```python
from build123d import *

# Parameters (mm, degrees)
F0_W      = 508
F0_H      = 254
F1_DEPTH  = 2.54
F3_DEPTH  = 203.2
F5_DEPTH  = 203.2
F6_W      = 76.2
F6_H      = 155.0987733221
F7_DEPTH  = 25.4
F9_DEPTH  = 76.2
F10_W     = 7.7724000598
F10_H     = 15.7987965533
F10_H_2   = 18.846809864
F10_H_3   = 19.9136117986
F11_DEPTH = 76.2
F12_W     = 38.3358041449
F12_H     = 114.723880429
F13_DEPTH = 25.4
F14_R     = 12.7
F15_DEPTH = 50.8
F16_W     = 76.2
F16_H     = 165.1
F17_DEPTH = 25.4
F18_W     = 254
F18_H     = 8.89
F18_W_2   = 139.9702800131
F19_DEPTH = 38.1


with BuildPart() as f1:
    # F0 (on Top) → F1 (new body)
    with BuildSketch(Plane.XY):
        with Locations((1.6115792096, -65.0062360242)):
            Rectangle(F0_W, F0_H)
    extrude(amount=F1_DEPTH)

    # F2 (on face) → F3 (join)
    with BuildSketch(Plane.XY.offset(2.54)):
        Polygon((-252.3884207904, 61.9937639758), (-252.3884207904, -192.0062360242), (-249.8484207904, -192.0062360242), (-249.8484207904, 59.4537639758), (255.6115792096, 59.4537639758), (255.6115792096, 61.9937639758), align=None)
    extrude(amount=F3_DEPTH)

    # F4 (on face) → F5 (join)
    with BuildSketch(Plane.XY.offset(2.54)):
        Polygon((-249.8484207904, -189.4662360242), (-249.8484207904, -192.0062360242), (-122.8484207904, -192.0062360242), (-139.9702800131, 59.4537639758), (-142.5102800131, 59.4537639758), (-125.5613688634, -189.4662360242), align=None)
    extrude(amount=F5_DEPTH)

    # F6 (on face) → F7 (cut)
    with BuildSketch(Plane(origin=(-135.2948289897, -9.2121968326, 0), x_dir=(-0.0679324996, 0.9976899195, 0), z_dir=(0.9976899195, 0.0679324996, 0))):
        with Locations((-38.1, 80.0893866611)):
            Rectangle(F6_W, F6_H)
    extrude(amount=-F7_DEPTH, mode=Mode.SUBTRACT)

    # F8 (on face) → F9 (join)
    with BuildSketch(Plane.XY.offset(2.54)):
        Polygon((-78.7540227175, -182.3542267084), (-43.1940241251, -182.3542267084), (-7.6340255328, -182.3542267084), (-28.2588265836, -108.7450310588), (-43.1940241251, -108.7450310588), (-58.1292216666, -108.7450310588), align=None)
    extrude(amount=F9_DEPTH)

    # F10 (on face) → F11 (join)
    with BuildSketch(Plane.XY.offset(2.54)):
        with Locations((-1.2078255029, -83.0656343008)):
            Rectangle(F10_W, F10_H)
        with Locations((-1.2078255029, -132.7480375767)):
            Rectangle(F10_W, F10_H_2)
        with Locations((-1.2078255029, -179.5094301249)):
            Rectangle(F10_W, F10_H_3)
        with Locations((29.1197744374, -83.0656343008)):
            Rectangle(F10_W, F10_H)
        with Locations((29.1197744374, -132.7480375767)):
            Rectangle(F10_W, F10_H_2)
        with Locations((29.1197744374, -179.5094301249)):
            Rectangle(F10_W, F10_H_3)
        Polygon((86.0411706011, -108.7450310588), (56.1707755181, -108.7450310588), (35.5459744672, -182.3542267084), (106.665971652, -182.3542267084), align=None)
    extrude(amount=F11_DEPTH)

    # F12 (on face) → F13 (join)
    with BuildSketch(Plane.XY.offset(78.74)):
        with Locations((14.0738765397, -132.5281762387)):
            Rectangle(F12_W, F12_H)
    extrude(amount=-F13_DEPTH)

    # F14 (on face) → F15 (join)
    with BuildSketch(Plane.XY.offset(2.54)):
        with Locations((-43.1940241251, -90.2538299561)):
            Circle(F14_R)
        with Locations((71.1059730596, -90.2538299561)):
            Circle(F14_R)
    extrude(amount=F15_DEPTH)

    # F16 (on face) → F17 (cut)
    with BuildSketch(Plane.XZ.offset(-59.4537639758)):
        with Locations((192.1115792096, 85.09)):
            Rectangle(F16_W, F16_H)
    extrude(amount=-F17_DEPTH, mode=Mode.SUBTRACT)

    # F18 (on face) → F19 (join)
    with BuildSketch(Plane.XZ.offset(-59.4537639758)):
        with Locations((-12.9702800131, 57.785)):
            Rectangle(F18_W, F18_H)
        with Locations((-12.9702800131, 104.775)):
            Rectangle(F18_W, F18_H)
        with Locations((-69.9851400065, 151.765)):
            Rectangle(F18_W_2, F18_H)
    extrude(amount=F19_DEPTH)


solid = f1.part
```
Work out the finished part from the listing and answer in its coordinate system (mm). A direction names the side the tool comes from. Give positions to 0.01 mm unless a question says otherwise; leave off trailing zeros. Loops run counter-clockwise (first coordinate to the right, second up) from the corner with the lowest first, then second, coordinate; pieces in that order, holes last. Notation, with made-up numbers: (36, 72.25) - (83, 72.25) arc R11 ccw to (83, 84.25) - close; hole circle Ø4 at (-13, -32). An arc over 180 degrees is marked (long way). Use CSV: the item, a comma, the result in double quotes. Start each with the question number.
(1) Each of these flat-tipped pins is pushed along its axis until it touches: pin 1 (11.5 mm diameter, centred on x = -30.5, y = 33, fed in from +Z); pin 2 (2.5 mm diameter, centred on y = 43.5, z = 104, fed in from +X); pin 3 (2 mm diameter, centred on y = -75.5, z = 162.5, fed in from +X). Where does it stop, or does it pass through?
(2) Find section C-C, the plane y = -59. Determine the outline of the cut face in (x, z), plus the area to 3 significant figures.
(3) Find section D-D, the plane x = -187. Determine the outline of the cut face in (y, z).
(4) Determine the mould class of faces 1 (the face through (2.678, -180, 28)), 2 (the face through (-15, 41, 109.22)) for opening direction X: released by +X, released by -X, zero draft, split by the parting line, or undercut.
(5) Find section B-B, the plane z = 117.5. Determine the outline of the cut face in (x, y).
(6) A tool of negligible diameter and unlimited length cuts with its end or side. For faces 3 (the face through (-45.95, -102.65, 27.58)), 4 (the face through (14, -189.89, 66)), 5 (the face through (14, -75.166, 58)), 6 (the face through (2.678, -133, 28)), from which of +Z, -Z, +X, -X, +Y, -Y can it reach the whole face along a straight path? Write none if from no direction.
(7) Find the intervals of material crossed by L1, parallel to Y at x = -174.5, z = 137; L2, parallel to X at y = -9.5, z = 185; L3, parallel to X at y = -156, z = 41.5, in increasing order.
(8) Find section A-A, the plane x = 173. Determine the outline of the cut face in (y, z).
Results found:
1,pin 1,"z = 156.21"
1,pin 2,"x = 114.03"
1,pin 3,"x = -130.71"
2,outline,"(-252.39, 0) - (255.61, 0) - (255.61, 2.54) - (-249.85, 2.54) - (-249.85, 205.74) - (-252.39, 205.74) - close; (-134.44, 157.64) - (-131.9, 157.64) - (-131.9, 205.74) - (-134.44, 205.74) - close"
2,area,"1,930 mm^2"
3,outline,"(-192.01, 0) - (61.99, 0) - (61.99, 205.74) - (59.45, 205.74) - (59.45, 2.54) - (-189.47, 2.54) - (-189.47, 205.74) - (-192.01, 205.74) - close"
4,face 1,"undercut"
4,face 2,"zero draft"
5,outline,"(-252.39, -192.01) - (-122.85, -192.01) - (-130.12, -85.24) - (-132.65, -85.41) - (-125.56, -189.47) - (-249.85, -189.47) - (-249.85, 59.45) - (-142.51, 59.45) - (-137.82, -9.38) - (-135.29, -9.21) - (-139.97, 59.45) - (154.01, 59.45) - (154.01, 61.99) - (-252.39, 61.99) - close; (230.21, 59.45) - (255.61, 59.45) - (255.61, 61.99) - (230.21, 61.99) - close"
6,face 3,"+Z"
6,face 4,"+Z, +X, -Y"
6,face 5,"+Z, +X"
6,face 6,"-Y"
7,L1,"-192.01 to -189.47, 59.45 to 61.99"
7,L2,"-252.39 to -249.85, -137.82 to -135.28"
7,L3,"-252.39 to -249.85, -127.84 to -125.3, -71.37 to -15.02, 42.93 to 99.28"
8,outline,"(-192.01, 0) - (61.99, 0) - (61.99, 2.54) - (-192.01, 2.54) - close; (59.45, 167.64) - (61.99, 167.64) - (61.99, 205.74) - (59.45, 205.74) - close"
